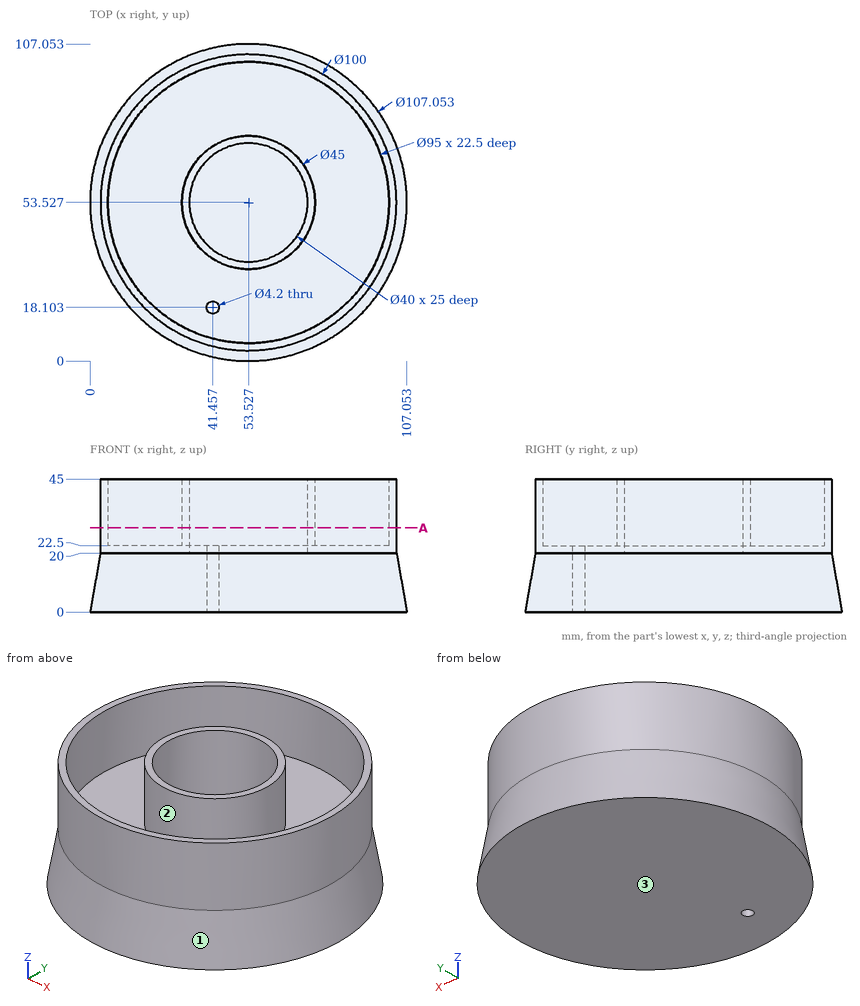
Input: dimensioned drawing with shaded views. Units: mm. Origin: part minimum x, y, z. Round coordinates to 2 decimals unless told otherwise and drop trailing zeros. Loops run counter-clockwise (first coordinate to the right, second up) from the corner with the lowest first, then second, coordinate; pieces in that order, holes last.
1) Material intervals for line 1 (Z direction, x = 26, y = 62); line 2 (Y direction, x = 93.5, z = 33.5) (1 decimal); line 3 (Y direction, x = 64.5, z = 23.5) (1 decimal), sorted ascending.
Ans:
line 1: z = 0 to 22.5
line 2: y = 23.5 to 27.9, 79.2 to 83.6
line 3: y = 4.7 to 7.3, 33.9 to 36.8, 70.2 to 73.2, 99.7 to 102.3
2) Section query A-A on z = 28.5. Return the cut outline in (x, y).
Ans:
outline: circle Ø100 at (53.53, 53.53); circle Ø45 at (53.53, 53.53); hole circle Ø95 at (53.53, 53.53); hole circle Ø40 at (53.53, 53.53)
3) Pin query (flat end, axial travel): pin 1 (3 mm diameter, centred on y = 40, z = 33, fed in from -X) (1 decimal); pin 2 (12 mm diameter, centred on x = 46, y = 76, fed in from +Z); pin 3 (8 mm diameter, centred on x = 75.5, z = 25, fed in from -Y); pin 4 (5 mm diameter, centred on x = 28, y = 37.5, fed in from +Z). Return the tip coordinate at first contact, or that it passes through.
Ans:
pin 1: stops at x = 5
pin 2: stops at z = 45
pin 3: stops at y = 6.87
pin 4: stops at z = 22.5
4) Pull-direction query (Y, two-part tool) for the marked faces 1, 2 and 3; classes: released by +Y, released by -Y, zero draft, split by the parting line, or undercut.
Ans:
face 1: split by the parting line
face 2: undercut
face 3: zero draft
